Design review of the part shown in the three views and the two pictorial views. Dimensions are in mm from the part's minimum x, y and z. Round coordinates to 2 decimals unless told otherwise and drop trailing zeros. Loops run counter-clockwise (first coordinate to the right, second up) from the corner with the lowest first, then second, coordinate; pieces in that order, holes last. Notation, with made-up numbers: (38, 37.5) - (65, 37.5) arc R13 ccw to (65, 58.5) - close; hole circle Ø2 at (69.25, 73.25). An arc over 180 degrees is marked (long way). Return JSON: item names as keys, results as strings. Group by question number.
(1) Clearance check with flat-ended pins moving along their axes: pin 1 (4 mm diameter, centred on x = 201.5, z = 4, fed in from -Y); pin 2 (4.5 mm diameter, centred on y = 263.5, z = 4.5, fed in from +X). State where each tip first meets the part, or that it passes through.
(2) Wall thickness on L1, parallel to Y at x = 69, z = 4.25; L2, parallel to Y at x = 266.5, z = 3.25; L3, parallel to X at y = 347.5, z = 5.5: over which ranges is each line inside the solid? List them lowest first. Write a range as [from, to].
(3) We need section A-A, the plane x = 264.5. Write out the cut boundary in (y, z).
(4) We need section D-D, the plane z = 4.5. Write out the cut boundary in (x, y), and give its area (3 significant figures).
(5) We need section C-C, the plane x = 110. Write out the cut boundary in (y, z).
(6) We need section B-B, the plane y = 27.5. Write out the cut boundary in (x, z).
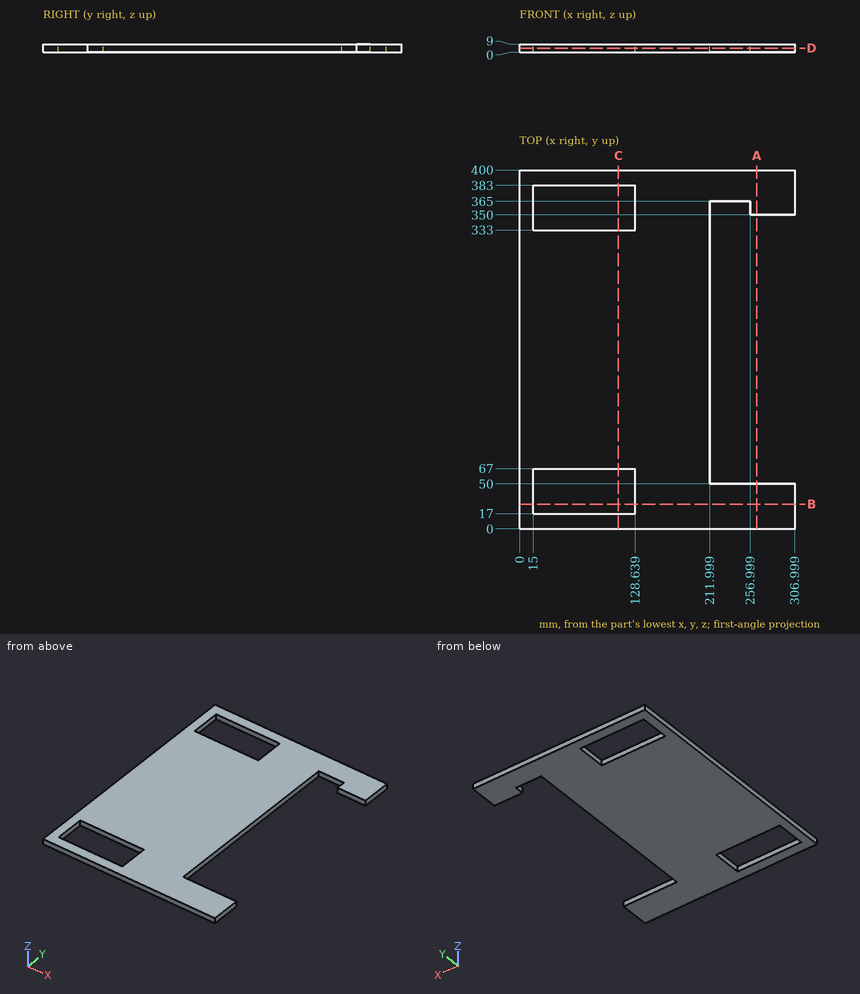
Solutions:
{
 "1": {"pin 1": "y = 0", "pin 2": "x = 212"},
 "2": {"L1": "[0, 17], [67, 333], [383, 400]", "L2": "[0, 50], [350, 400]", "L3": "[0, 15], [128.64, 212]"},
 "3": {"outline": "(0, 0) - (50, 0) - (50, 9) - (0, 9) - close; (350, 0) - (400, 0) - (400, 9) - (350, 9) - close"},
 "4": {"outline": "(0, 0) - (307, 0) - (307, 50) - (212, 50) - (212, 365) - (257, 365) - (257, 350) - (307, 350) - (307, 400) - (0, 400) - close; hole (15, 17) - (128.64, 17) - (128.64, 67) - (15, 67) - close; hole (15, 333) - (128.64, 333) - (128.64, 383) - (15, 383) - close", "area": "82,300 mm^2"},
 "5": {"outline": "(0, 0) - (17, 0) - (17, 9) - (0, 9) - close; (67, 0) - (333, 0) - (333, 9) - (67, 9) - close; (383, 0) - (400, 0) - (400, 9) - (383, 9) - close"},
 "6": {"outline": "(0, 0) - (15, 0) - (15, 9) - (0, 9) - close; (128.64, 0) - (307, 0) - (307, 9) - (128.64, 9) - close"}
}
